Study the drawing (mm; zero at the part's minimum x, y, z) and answer. Round coordinates to 2 decimals unless told otherwise and drop trailing zeros. Loops run counter-clockwise (first coordinate to the right, second up) from the corner with the lowest first, then second, coordinate; pieces in that order, holes last. Notation, with made-up numbers: (-6, 49.5) - (-2, 49.5) arc R6 ccw to (-2, 56.5) - close; hole circle Ø5 at (36.25, 32.25). An arc over 180 degrees is marked (long way). One line per item, written item: value.
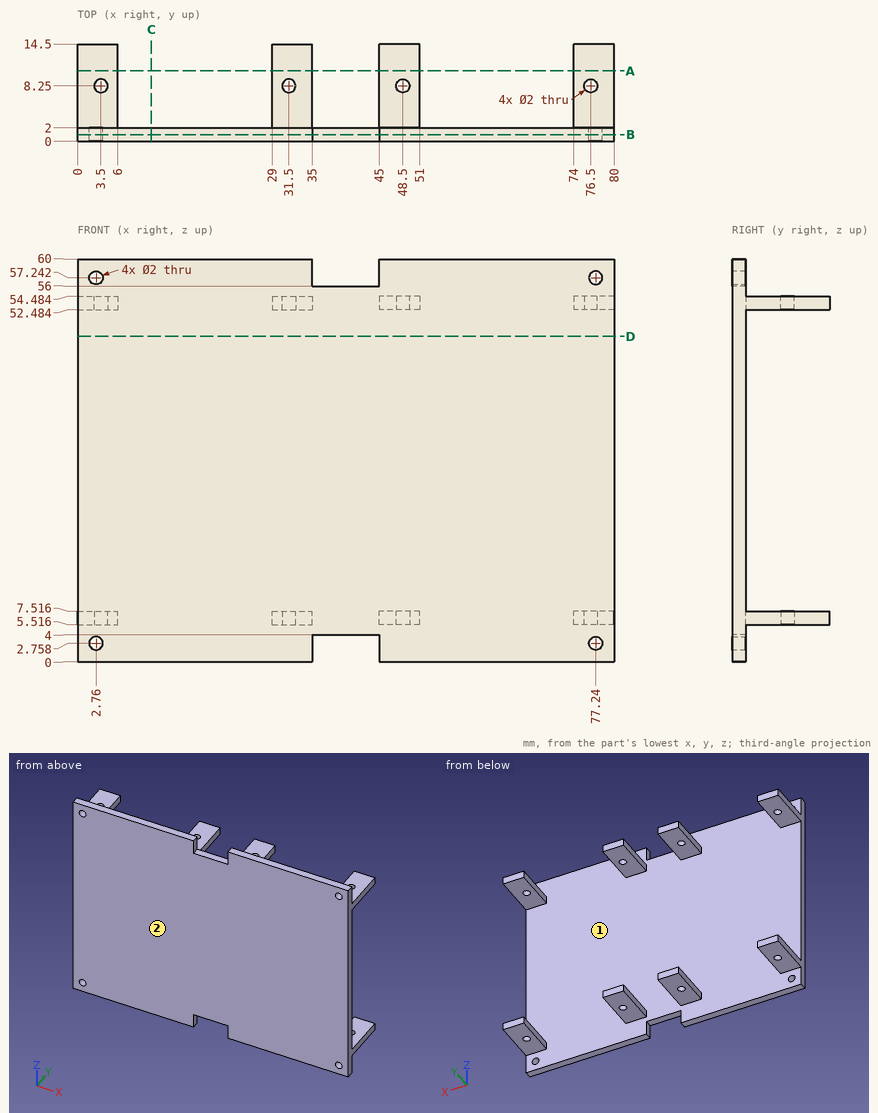
1) A cutting plane is placed at D-D on z = 48.5. Give the vertices of the cut face in (x, y).
Final values:
outline: (0, 0) - (80, 0) - (80, 2) - (0, 2) - close
2) Consider L1, parallel to X at y = 10.25, z = 6.5; L2, parallel to Z at x = 30.5, y = 12.25; L3, parallel to Y at x = 48.5, z = 53.85. Determine where each line is inside the solid, lowest interval first.
Final values:
L1: 0 to 6, 29 to 35, 45 to 51, 74 to 80
L2: 5.52 to 7.52, 52.48 to 54.48
L3: 0 to 7.25, 9.25 to 14.5
3) Each of these flat-tipped pins is pushed along its axis until it touches: pin 1 Ø2.5 at (x, y) = (3.5, 8.25) entering from +Z; pin 2 Ø1.8 at (x, y) = (47.5, 5) entering from -Z; pin 3 Ø2 at (x, y) = (41.5, 1) entering from -Z; pin 4 Ø1.6 at (x, z) = (2.76, 57.24) entering from +Y. Where does it stop, or does it pass through?
Final values:
pin 1: z = 54.48
pin 2: z = 5.52
pin 3: z = 4
pin 4: through
4) A cutting plane is placed at B-B on y = 1. Give the vertices of the cut face in (x, z), and give its area (3 significant figures).
Final values:
outline: (0, 0) - (35, 0) - (35, 4) - (45, 4) - (45, 0) - (80, 0) - (80, 60) - (45, 60) - (45, 56) - (35, 56) - (35, 60) - (0, 60) - close; hole circle Ø2 at (2.76, 2.76); hole circle Ø2 at (2.76, 57.24); hole circle Ø2 at (77.24, 2.76); hole circle Ø2 at (77.24, 57.24)
area: 4,710 mm2
5) For a pull along Z with two mould halves and no side action, classify the marked faces 1 and 2 as released by +Z, released by -Z, zero draft, split by the parting line, or undercut.
Final values:
face 1: undercut
face 2: zero draft
6) A cutting plane is placed at A-A on y = 10.5. Give the number of separate pieces and of enclosed holes in the cut face.
Final values:
separate pieces: 8
enclosed holes: 0
7) A cutting plane is placed at C-C on x = 11. Give the vertices of the cut face in (y, z).
Final values:
outline: (0, 0) - (2, 0) - (2, 60) - (0, 60) - close
